Work out the finished part from the listing and answer in its coordinate system (mm). A direction names the side the tool comes from. Coordinates: 2 decimals unless noted, no trailing zeros. Loops run counter-clockwise (first coordinate to the right, second up) from the corner with the lowest first, then second, coordinate; pieces in that order, holes last. Notation, with made-up numbers: (-1.5, -1) -> (2.5, -1) arc R9 cw to (2.5, 15) -> close; hole circle Ø11 at (10.5, 45). An arc over 180 degrees is marked (long way). One line per question, with ' | ' between items.
```python
from build123d import *

# Parameters (mm, degrees)
EXTRUDE1_DEPTH = 68
FILLET1_R      = 1
EXTRUDE2_DEPTH = 7.5
CHAMFER1_SIZE  = 1.5
CHAMFER2_SIZE  = 0.5


with BuildPart() as part:
    # Sketch1 → Revolve1 (revolve)
    with BuildSketch(Plane.XY, mode=Mode.PRIVATE) as revolve1_sk:
        Polygon((0, 0), (297, 0), (297, 37.5), (177, 37.5), (177, 39.5), (142, 39.5), (142, 40), (105, 40), (105, 49), (37, 49), (37, 40), (0, 40), align=None)
    revolve(revolve1_sk.sketch.rotate(Axis((0, 0, 0), (-1, 0, 0)), 90), axis=Axis((0, 0, 0), (-1, 0, 0)))

    # Sketch2 → Extrude1 (cut)
    with BuildSketch(Plane.ZY.offset(-37)):
        with BuildLine():
            Line((-10, 47.968739821), (-10, 41.5))
            Line((-10, 41.5), (10, 41.5))
            Line((10, 41.5), (10, 47.968739821))
            ThreePointArc((10, 47.968739821), (0, 49), (-10, 47.968739821))
        make_face()
        with BuildLine():
            Line((-47.968739821, 10), (-41.5, 10))
            Line((-41.5, 10), (-41.5, -10))
            Line((-41.5, -10), (-47.968739821, -10))
            ThreePointArc((-47.968739821, -10), (-49, 0), (-47.968739821, 10))
        make_face()
    extrude(amount=-EXTRUDE1_DEPTH, mode=Mode.SUBTRACT)

    # Fillet1
    fillet1_edges = [part.edges().sort_by_distance(p)[0] for p in [
        (177, 0, 37.5),
        (105, 0, 40),
        (37, 0, 40),
    ]]
    fillet(fillet1_edges, radius=FILLET1_R)

    # Sketch3 → Extrude2 (cut)
    with BuildSketch(Plane(origin=(237.5, 37.5, 0), x_dir=(0, 0, 1), z_dir=(0, 1, 0))):
        with BuildLine():
            Line((-10, 59.5), (-10, -40.5))
            ThreePointArc((-10, -40.5), (0, -50.5), (10, -40.5))
            Line((10, -40.5), (10, 59.5))
            ThreePointArc((10, 59.5), (0, 69.5), (-10, 59.5))
        make_face()
    extrude(amount=-EXTRUDE2_DEPTH, mode=Mode.SUBTRACT)

    # Chamfer1
    chamfer1_edges = [part.edges().sort_by_distance(p)[0] for p in [
        (0, 0, 40),
        (297, -29.843340966, 22.707377656),
    ]]
    chamfer(chamfer1_edges, length=CHAMFER1_SIZE)

    # Chamfer2
    chamfer2_edges = [part.edges().sort_by_distance(p)[0] for p in [
        (105, -34.648232278, 34.648232278),
        (37, -34.648232278, 34.648232278),
        (105, 34.648232278, -34.648232278),
        (37, 34.648232278, -34.648232278),
    ]]
    chamfer(chamfer2_edges, length=CHAMFER2_SIZE)


solid = part.part
```
1) Find the intervals of material crossed by line 1 along Z through (x, y) = (148, 9); line 2 along Y through (x, z) = (178.5, 2); line 3 along Z through (x, y) = (136, 14), in increasing order.
Check values:
line 1: z = -38.46 to 38.46 | line 2: y = -37.45 to 37.45 | line 3: z = -37.47 to 37.47
2) The mould has two halves that part along Y. Classify faces 4 (the face through (243, 30, 0)), 5 (the face through (248, 33, -10)), 6 (the face through (71, 10, -45)): released by +Y, released by -Y, zero draft, split by the parting line, or undercut.
Check values:
face 4: released by +Y | face 5: zero draft | face 6: undercut
3) For faces 1 (the face through (159.255, -11.865, -37.676)), 2 (the face through (18.51, -1.76, 39.96)), 3 (the face through (246, 33, 10)), determine the directions among +Z, -Z, +X, -X, +Y, -Y from which every point of the face is accessible in a straight line to the end or side of a thin tool.
Check values:
face 1: +X | face 2: -X | face 3: +X, +Y
4) Find section C-C (x = 162). Write down the section's boundary in (y, z).
Check values:
outline: circle Ø79 at (0, 0)
5) Flat-ended cylindrical pins translate along their axes: pin 1 (5 mm diameter, centred on x = 61.5, y = 44, fed in from +Z); pin 2 (6 mm diameter, centred on x = 67, z = 21.5, fed in from +Y); pin 3 (7 mm diameter, centred on x = 80.5, z = -46, fed in from -Y). Find the tip coordinate at first contact, or state that the pin passes through.
Check values:
pin 1: stops at z = 26.05 | pin 2: stops at y = 45.37 | pin 3: stops at y = -24.39
